```python
from build123d import *

# Parameters (mm, degrees)
F0_W     = 30.48
F0_H     = 5.08
F0_W_2   = 2.54
F1_DEPTH = 0.635
F0_H_2   = 6.985
F2_DEPTH = 0.635


with BuildPart() as f1:
    # F0 (on Front) → F1 (new body, symmetric)
    with BuildSketch(Plane.XZ):
        Polygon((-109.3809070776, 2.54), (-109.3809070776, -2.54), (43.9970903099, -2.54), (60.7990929224, 0), (43.9970903099, 2.54), align=None)
        with Locations((-127.1609070776, 0)):
            Rectangle(F0_W, F0_H)
        with Locations((-110.6509070776, 0)):
            Rectangle(F0_W_2, F0_H)
    extrude(amount=F1_DEPTH, both=True)

    # F0 (on Front) → F2 (join, symmetric)
    with BuildSketch(Plane.XZ):
        with Locations((-110.6509070776, 6.0325)):
            Rectangle(F0_W_2, F0_H_2)
        with Locations((-110.6509070776, -6.0325)):
            Rectangle(F0_W_2, F0_H_2)
    extrude(amount=F2_DEPTH, both=True)


solid = f1.part
```
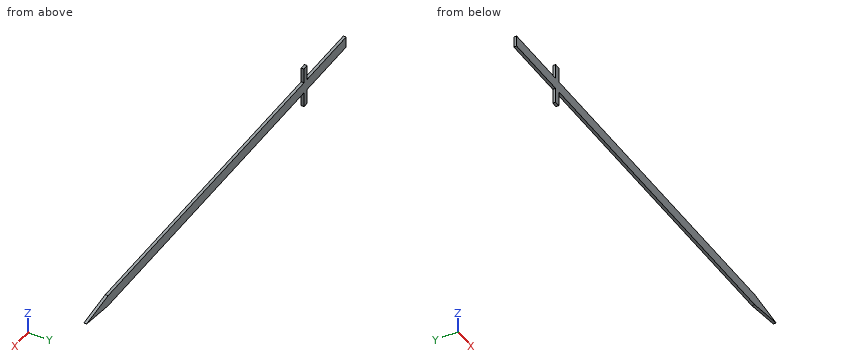
Can you work these out from the model? Positions are in its coordinate system, mm. Round coordinates to 2 decimals unless told otherwise and drop trailing zeros. Order: outer loops, then holes, each group sorted by start corner. A loop starts at its lowest first (then second) coordinate and runs counter-clockwise, first axis right, second up. Notation, with made-up numbers: (80.5, 57) -> (104.5, 57) arc R21 ccw to (104.5, 78) -> close; hole circle Ø6 at (-36, 11). An arc over 180 degrees is marked (long way). Return JSON: item names as keys, results as strings. Group by question number.
1. If we section it at C-C, the plane z = -7: Write out the boundary of the cut face in (x, y) (3 decimals), then the cut area to 3 significant figures.
2. I need wall thicknesses on line 1 (X direction, y = -0.15, z = 7.25); line 2 (Z direction, x = -120, y = -0.4). Which ranges of each line are inside material? Lowest first, please. Write a range as [from, to].
3. If we section it at B-B, the plane x = -96: Write out the boundary of the cut face in (y, z) (3 decimals).
4. Will these pins go through, and if not, where does the flat tip stop? pin 1 (0.6 mm diameter, centred on y = 0.5, z = 7.5, fed in from +X); pin 2 (0.6 mm diameter, centred on x = -69, y = 0.5, fed in from +Z).
5. If we section it at A-A, the plane y = -0.1: Write out the boundary of the cut face in (x, z) (3 decimals), then the cut area to 3 significant figures.
Output values:
{
 "1": {"outline": "(-111.921, -0.635) -> (-109.381, -0.635) -> (-109.381, 0.635) -> (-111.921, 0.635) -> close", "area": "3.23 mm²"},
 "2": {"line 1": "[-111.92, -109.38]", "line 2": "[-2.54, 2.54]"},
 "3": {"outline": "(-0.635, -2.54) -> (0.635, -2.54) -> (0.635, 2.54) -> (-0.635, 2.54) -> close"},
 "4": {"pin 1": "x = -109.38", "pin 2": "z = 2.54"},
 "5": {"outline": "(-142.401, -2.54) -> (-111.921, -2.54) -> (-111.921, -9.525) -> (-109.381, -9.525) -> (-109.381, -2.54) -> (43.997, -2.54) -> (60.799, 0) -> (43.997, 2.54) -> (-109.381, 2.54) -> (-109.381, 9.525) -> (-111.921, 9.525) -> (-111.921, 2.54) -> (-142.401, 2.54) -> close", "area": "1,030 mm²"}
}
